Autodesk Fusion 360 part; units mm, degrees
sketch "Sketch1" plane through (0, 0, 0) normal (0, 1, 0) x (1, 0, 0)
  line L0 (0, 0) -> (0, -45)
  line L1 (0, -45) -> (15, -45)
  line L2 (15, -45) -> (15, -15)
  line L3 (15, -15) -> (75, -15)
  line L4 (75, -15) -> (75, 0)
  line L5 (75, 0) -> (0, 0)
  dimension "d1" = 45
  dimension "d2" = 15
  dimension "d3" = 30
  dimension "d4" = 60
extrude "Extrude1" add sketch "Sketch1" along normal blind 60
sketch "Sketch2" plane through (15, 0, 0) normal (1, 0, 0) x (0, 1, 0)
  line L0 (0, 45) -> (0, 15)
  line L1 (0, 15) -> (60, 15)
  line L2 (60, 15) -> (60, 45)
  line L3 (60, 45) -> (0, 45)
  circle A0 centre (11.5393, 30) radius 8
  circle A1 centre (46.5393, 30) radius 8
  dimension "d7" = 15
  dimension "d8" = 15
  dimension "d9" = 35
  dimension "d10" = 16
  dimension "d11" = 16
extrude "Extrude2" cut sketch "Sketch2" against normal blind 5 contours A0 | A1
sketch "Sketch3" plane through (0, 0, 15) normal (0, 0, 1) x (-1, 0, 0)
  line L0 (-15, 0) -> (-75, 0)
  line L1 (-75, 0) -> (-75, -60)
  line L2 (-75, -60) -> (-15, -60)
  line L3 (-15, -60) -> (-15, 0)
  line L4 (0, 0) -> (0, -30) construction
  line L5 (0, -30) -> (-75, -30) construction
  circle A0 centre (-75, -30) radius 30
  circle A1 centre (-75, -30) radius 20
  dimension "d14" = 30
  dimension "d15" = 75
  dimension "d16" = 60
  dimension "d17" = 40
extrude "Extrude4" cut sketch "Sketch3" against normal blind 60 contours L1 A0 A1 | L1 A0 A1 | L1 A1 | L1 A1
extrude "Extrude5" add sketch "Sketch3" along normal blind 0 and the other way blind 15 contours L1 A0 A1 | L1 A0 A1
extrude "Extrude6" add sketch "Sketch3" against normal blind 15 from surface at -15 contours L1 A0 A1 | L1 A0 A1
extrude "Extrude7" add sketch "Sketch3" along normal blind 30 contours L1 A0 A1 | L1 A0 A1
sketch "Sketch4" plane through (0, 0, 0) normal (0, -1, 0) x (1, 0, 0)
  line L0 (0, 0) -> (75, 0)
  line L1 (75, 0) -> (75, 15)
  line L2 (75, 15) -> (15, 15)
  line L3 (15, 15) -> (15, 45)
  line L4 (15, 45) -> (0, 45)
  line L5 (0, 45) -> (0, 0)
sketch "Sketch5" plane through (0, 0, 45) normal (0, 0, 1) x (-1, 0, 0)
  circle A0 centre (-75, -30) radius 20
  circle A1 centre (-75, -30) radius 30
sketch "Sketch6" plane through (0, 0, 0) normal (-1, 0, 0) x (0, -1, 0)
  line L0 (0, 0) -> (0, 45)
  line L1 (0, 45) -> (-60, 45)
  line L2 (-60, 45) -> (-60, 0)
  line L3 (-60, 0) -> (0, 0)
sketch "Sketch7" plane through (0, 0, 0) normal (-1, 0, 0) x (0, -1, 0)
sketch "Sketch8" plane through (0, 0, 0) normal (0, -1, 0) x (1, 0, 0)
sketch "Sketch9" plane through (0, 0, 45) normal (0, 0, 1) x (-1, 0, 0)
sketch "Sketch10" plane through (0, 0, 0) normal (0, 0, -1) x (1, 0, 0)
  arc A0 (75, 0) -> (75, -60) centre (75, -30) ccw
  line L0 (75, 0) -> (0, 0)
  line L1 (0, 0) -> (0, -60)
  line L2 (0, -60) -> (75, -60)
  circle A1 centre (75, -30) radius 30
  circle A2 centre (75, -30) radius 20
  line L3 (75, 0) -> (150, 0)
  line L4 (150, 0) -> (150, -60)
  line L5 (150, -60) -> (75, -60)
extrude "Extrude8" add sketch "Sketch10" along normal blind 15 contours A1 L3 L4 L5
fillet "Fillet1" radius 25 2 edges at (150, 60, -7.5) (150, 0, -7.5)
sketch "Sketch11" plane through (0, 0, 45) normal (0, 0, 1) x (-1, 0, 0)
  line L0 (0, 0) -> (-15, 0)
  line L1 (-15, 0) -> (-15, -60)
  line L2 (-15, -60) -> (0, -60)
  line L3 (0, -60) -> (0, 0)
Geometry: final body of the model. Coordinates: model frame, mm. A direction names the side the tool comes from. Round coordinates to 2 decimals unless told otherwise and drop trailing zeros. Loops run counter-clockwise (first coordinate to the right, second up) from the corner with the lowest first, then second, coordinate; pieces in that order, holes last. Notation, with made-up numbers: M 24,44.25 L 82,44.25 A24 cw 82,75.25 Z; hole C 61.5,70 d6. An arc over 180 degrees is marked long. Put each result on its own line as item: value. Start each with the question number.
(1) Section query C-C (z = 2.5). Return loops of the section in (x, y).
(2) Set-up query: faces 5 (the face through (108, 30, -15)), 6 (the face through (45.007, 30.66, -7.395)), 7 (the face through (12.54, 54.17, 32.4)), 8 (the face through (15, 30, 30)). Return all of +Z, -Z, +X, -X, +Y, -Y with unobstructed straight access to the full face (end or side cutting, diameter ignored); none if empty.
(3) Section query D-D (y = 13). Return loops of the section in (x, z).
(4) Material intervals for line 1 along X through (y, z) = (30, 20); line 2 along Y through (x, z) = (75, 19); line 3 along X through (y, z) = (20.5, 18.5), sorted ascending. Write a range as [from, to].
(5) Draft query along Z for faces 1 (the face through (0, 30, 22)), 2 (the face through (12.535, 15.84, 36.746)), 3 (the face through (10, 11, 30)), 4 (the face through (69, 50, 45)). Return one class per face: +Z half, -Z half, draft (parallel to the pull), parting line (faces both ways), or undercut.
(6) Section query B-B (y = 30). Return loops of the section in (x, z).
(7) Contact query for flat-ended pins moving along their axis: pin 1 Ø1.5 at (y, z) = (25.5, 29) entering from -X; pin 2 Ø13 at (y, z) = (46, 29.5) entering from +X; pin 3 Ø4 at (y, z) = (30, -4) entering from -X; pin 4 Ø8 at (y, z) = (7.5, 27) entering from +X. Output: stop coordinate, or through.
(8) Section query A-A (z = 30). Return loops of the section in (x, y), then the cut area to 3 significant figures.
Findings below:
1. outline: M 0,0 L 75,0 A30 ccw 75,60 L 0,60 Z; hole C 75,30 d40
2. face 5: -Z, +X, -X, +Y, -Y
2. face 6: -Z, -X
2. face 7: none
2. face 8: +Z, +Y, -Y
3. outline: M 0,0 L 50.28,0 L 50.28,-15 L 64.46,-15 L 64.46,45 L 50.28,45 L 50.28,15 L 15,15 L 15,22.13 L 10,22.13 L 10,37.87 L 15,37.87 L 15,45 L 0,45 Z; M 85.54,-15 L 146.93,-15 L 146.93,0 L 99.72,0 L 99.72,45 L 85.54,45 Z
4. line 1: x = [0, 15], [45, 55], [95, 105]
4. line 2: y = [0, 10], [50, 60]
4. line 3: x = [0, 15], [46.54, 57.4], [92.6, 103.46]
5. face 1: draft
5. face 2: undercut
5. face 3: undercut
5. face 4: +Z half
6. outline: M 0,0 L 45,0 L 45,-15 L 55,-15 L 55,45 L 45,45 L 45,15 L 15,15 L 15,45 L 0,45 Z; M 95,-15 L 150,-15 L 150,0 L 105,0 L 105,45 L 95,45 Z
7. pin 1: stops at x = 0
7. pin 2: stops at x = 103.46
7. pin 3: stops at x = 45
7. pin 4: stops at x = 98.62
8. outline: M 0,0 L 15,0 L 15,3.54 L 10,3.54 L 10,19.54 L 15,19.54 L 15,38.54 L 10,38.54 L 10,54.54 L 15,54.54 L 15,60 L 0,60 Z; C 75,30 d60; hole C 75,30 d40
8. area: 2,310 mm2
